from build123d import *


with BuildPart() as part:
    # Çizim1 → Döndür1 (revolve)
    with BuildSketch(Plane(origin=(0, 0, 0), x_dir=(1, 0, 0), z_dir=(0, 1, 0)), mode=Mode.PRIVATE) as d_nd_r1_sk:
        Polygon((0, 0), (0, -138.2), (3.5, -138.2), (3.5, -130.78), (4, -130.78), (4, -121.38), (5, -121.38), (5, -116.38), (10, -116.38), (10, -36.38), (5, -36.38), (5, -32.88), (4, -32.88), (4, 0), align=None)
    revolve(d_nd_r1_sk.sketch.rotate(Axis((0, 0, 0), (0, 0, 1)), 180), axis=Axis((0, 0, 0), (0, 0, 1)))


solid = part.part
Geometry check sheet. Reference: the model listing, model coordinates, mm. A direction names the side the tool comes from. Round coordinates to 2 decimals unless told otherwise and drop trailing zeros. Order: outer loops, then holes, each group sorted by start corner. A loop starts at its lowest first (then second) coordinate and runs counter-clockwise, first axis right, second up. Notation, with made-up numbers: (39, -35) - (65, -35) arc R16 ccw to (65, -8) - close; hole circle Ø9 at (1, 75). An arc over 180 degrees is marked (long way). One line per question, with ' | ' between items. Start each with the question number.
(1) Sectioned sample at A-A on y = 0. Record the cut outline in (x, z), and give its area (3 significant figures).
(2) Depth check by flat-ended pin: pin 1 Ø1 at (x, z) = (4, 63) entering from -Y; pin 2 Ø1.5 at (x, y) = (-6, 0.5) entering from -Z; pin 3 Ø1.5 at (y, z) = (-6.5, 86.5) entering from -X. Enter the tip coordinate at first touch or a pass-through.
(3) Access from +Z, -Z, +X, -X, +Y, -Y to the whole of each face (thin tool, end or side, straight path). Record for faces 1 (the cylindrical face through (5, 0, 35)), 2 (the cylindrical face through (-3.233, 1.341, 134.438)), 3 (the flat face through (0, 0, 0)).
(4) Thickness scan on L1, parallel to Z at x = -8.75, y = -3.5; L2, parallel to Y at x = -5.75, z = 40.5; L3, parallel to Y at x = -6.5, z = 107. Record the ranges inside material, lowest first. Write a range as [from, to].
(5) Sectioned sample at D-D on x = -6.5. Record the cut outline in (y, z).
(6) Sectioned sample at C-C on z = 63.5. Record the cut outline in (x, y).
Conclusion:
1) outline: (-10, 36.38) - (-5, 36.38) - (-5, 32.88) - (-4, 32.88) - (-4, 0) - (4, 0) - (4, 32.88) - (5, 32.88) - (5, 36.38) - (10, 36.38) - (10, 116.38) - (5, 116.38) - (5, 121.38) - (4, 121.38) - (4, 130.78) - (3.5, 130.78) - (3.5, 138.2) - (-3.5, 138.2) - (-3.5, 130.78) - (-4, 130.78) - (-4, 121.38) - (-5, 121.38) - (-5, 116.38) - (-10, 116.38) - close | area: 2,080 mm2
2) pin 1: stops at y = -9.37 | pin 2: stops at z = 36.38 | pin 3: stops at x = -8.18
3) face 1: -Z | face 2: +Z | face 3: -Z, +X, -X, +Y, -Y
4) L1: z = [36.38, 116.38] | L2: y = [-8.18, 8.18] | L3: y = [-7.6, 7.6]
5) outline: (-7.6, 36.38) - (7.6, 36.38) - (7.6, 116.38) - (-7.6, 116.38) - close
6) outline: circle Ø20 at (0, 0)
